Autodesk Inventor part; units mm, degrees
ref_plane "YZ Plane" through (0, 0, 0) normal (1, 0, 0) x (0, 1, 0)
ref_plane "XZ Plane" through (0, 0, 0) normal (0, 1, 0) x (-1, 0, 0)
ref_plane "XY Plane" through (0, 0, 0) normal (0, 0, 1) x (1, 0, 0)
sketch "Sketch1" plane through (0, 0, 0) normal (0, 0, 1) x (1, 0, 0)
  line L0 (0, 0) -> (75, 0)
  line L1 (75, 0) -> (75, 150)
  line L2 (75, 150) -> (0, 150)
  line L3 (0, 150) -> (0, 0)
  dimension "d0" = 75
  dimension "d1" = 150
extrude "Extrusion1" add sketch "Sketch1" along normal blind 10
sketch "Sketch2" plane through (0, 0, 10) normal (0, 0, 1) x (1, 0, 0)
  line L0 (17, 90) -> (17, 14)
  line L1 (17, 14) -> (27, 14)
  line L2 (27, 14) -> (27, 19)
  line L3 (27, 19) -> (22, 19)
  line L4 (22, 19) -> (22, 85)
  line L5 (22, 85) -> (27, 85)
  line L6 (27, 85) -> (27, 90)
  line L7 (27, 90) -> (17, 90)
  line L8 (75, 0) -> (75, 150)
  line L9 (75, 150) -> (0, 150)
  point P0 (0, 0)
  dimension "d4" = 76
  dimension "d5" = 10
  dimension "d6" = 5
  dimension "d7" = 66
  dimension "d8" = 53
  dimension "d9" = 5
  dimension "d10" = 60
extrude "Extrusion2" add sketch "Sketch2" along normal blind 5
sketch "Sketch3" plane through (22, 19, 10) normal (1, 0, 0) x (0, 0, -1)
  line L0 (-5, 0) -> (-5, 66)
  line L1 (-5, 66) -> (-3, 66)
  line L2 (-3, 66) -> (-3, 56)
  line L3 (-3, 56) -> (-5, 56)
  line L4 (-5, 56) -> (-5, 66)
  line L5 (-5, 0) -> (-3, 0)
  line L6 (-3, 0) -> (-3, 10)
  line L7 (-3, 10) -> (-5, 10)
  line L8 (-5, 10) -> (-5, 0)
  point P0 (10, -19)
  point P1 (-5, 10)
  point P2 (-5, 56)
  dimension "d13" = 2
  dimension "d14" = 10
  dimension "d15" = 10
  dimension "d73" = 2
extrude "Extrusion3" add sketch "Sketch3" along normal blind 3
sketch "Sketch4" plane through (0, 0, 10) normal (0, 0, 1) x (1, 0, 0)
  line L0 (75, 0) -> (75, 150)
  line L1 (75, 140) -> (10, 140)
  line L2 (10, 140) -> (10, 10)
  line L3 (10, 10) -> (75, 10)
  line L4 (75, 150) -> (0, 150)
  line L5 (0, 150) -> (0, 0)
  line L6 (0, 0) -> (75, 0)
  dimension "d18" = 10
  dimension "d19" = 10
  dimension "d20" = 10
extrude "Extrusion4" add sketch "Sketch4" along normal blind 140 contours L6 L5 L4 L0 L1 L2 L3
sketch "Sketch5" plane through (0, 0, 0) normal (-1, 0, 0) x (0, 0, 1)
  line L0 (90.0447, 124.5126) -> (90.0447, 94.5126)
  line L1 (90.0447, 94.5126) -> (109.0447, 94.5126)
  line L2 (109.0447, 94.5126) -> (109.0447, 64.5126)
  line L3 (109.0447, 64.5126) -> (90.0447, 64.5126)
  line L4 (90.0447, 64.5126) -> (90.0447, 77.5126)
  line L5 (90.0447, 77.5126) -> (76.4377, 86.2941)
  line L6 (76.4377, 86.2941) -> (46.4377, 86.2941)
  line L7 (46.4377, 86.2941) -> (46.4377, 56.2941)
  line L8 (46.4377, 56.2941) -> (65.4377, 56.2941)
  line L9 (65.4377, 56.2941) -> (65.4377, 37.2941)
  line L10 (65.4377, 37.2941) -> (77.4951, 29.5126)
  line L11 (77.4951, 29.5126) -> (118.4951, 29.5126)
  line L12 (118.4951, 29.5126) -> (135, 48.5)
  line L13 (135, 48.5) -> (135, 111.5)
  line L14 (135, 111.5) -> (120.0447, 124.5)
  line L15 (120.0447, 124.5) -> (90.0447, 124.5126)
  line L16 (0, 0) -> (150, 0)
  line L17 (150, 150) -> (150, 0)
  line L18 (36.4377, 86) -> (17.4377, 86)
  line L19 (17.4377, 86) -> (17.4377, 56)
  line L20 (17.4377, 56) -> (36.4377, 56)
  line L21 (36.4377, 56) -> (36.4377, 86)
  line L22 (10, 140) -> (150, 140)
  circle A0 centre (140, 140) radius 7.5
  line L23 (10, 10) -> (150, 10)
  circle A1 centre (140, 10) radius 7.5
  circle A2 centre (10, 140) radius 7.5
  line L24 (10, 10) -> (10, 140)
  circle A3 centre (10, 10) radius 7.5
  point P0 (99.5447, 64.5126)
  point P1 (135, 80)
  point P2 (26.9377, 56)
  dimension "d43" = 30
  dimension "d44" = 19
  dimension "d45" = 30
  dimension "d46" = 13
  dimension "d47" = 30
  dimension "d48" = 30
  dimension "d49" = 19
  dimension "d50" = 19
  dimension "d51" = 41
  dimension "d52" = 63
  dimension "d53" = 13
  dimension "d56" = 35
  dimension "d57" = 95
  dimension "d58" = 30
  dimension "d59" = 80
  dimension "d60" = 25.9553
  dimension "d61" = 15
  dimension "d62" = 19
  dimension "d63" = 10
  dimension "d67" = 15
  dimension "d68" = 15
  dimension "d69" = 15
  dimension "d70" = 15
  dimension "d71" = 10
  dimension "d72" = 10
  dimension "d112" = 56
  dimension "d113" = 30
extrude "Extrusion5" add sketch "Sketch5" along normal blind 3 contours L15 L14 L13 L12 L11 L10 L9 L8 L7 L6 L5 L4 L3 L2 L1 L0 | A0 L22 | L22 A0 | A1 L23 | L23 A1 | A2 L24 L22 | L22 L24 A2 | A3 L24 L23 | L23 L24 A3 | L21 L20 L19 L18
sketch "Sketch8" plane through (10, 10, 10) normal (0, 1, 0) x (1, 0, 0)
  line L0 (65, 0) -> (65, -140)
  line L1 (65, -115) -> (15, -115)
  line L2 (15, -115) -> (15, -85)
  line L3 (15, -85) -> (65, -85)
  line L4 (65, -115) -> (65, -120)
  line L5 (65, -120) -> (10, -120)
  line L6 (10, -120) -> (10, -80)
  line L7 (10, -80) -> (65, -80)
  line L8 (-10, -140) -> (65, -140)
  point P0 (-10, 10)
  dimension "d74" = 30
  dimension "d75" = 50
  dimension "d76" = 5
  dimension "d77" = 55
  dimension "d78" = 40
  dimension "d111" = 20
extrude "Extrusion6" add sketch "Sketch8" along normal blind 10 contours L0 L3 L2 L1 L5 L6 L7
sketch "Sketch10" plane through (25, 10, 125) normal (0, 1, 0) x (1, 0, 0)
  line L0 (50, 30) -> (50, 0)
  line L1 (0, 30) -> (50, 30)
  line L2 (50, 0) -> (0, 0)
  line L3 (0, 0) -> (0, 30)
  line L4 (0, 30) -> (50, 30)
  line L5 (50, 30) -> (50, 0)
  point P0 (-25, 125)
extrude "Extrusion7" cut sketch "Sketch10" against normal blind 10
sketch "Sketch11" plane through (25, 0, 95) normal (1, 0, 0) x (0, 0, -1)
  line L0 (85, 10) -> (-55, 10)
  line L1 (-29.957, 10) -> (0.043, 10)
  line L2 (0.043, 10) -> (0.043, 13)
  line L3 (0.043, 13) -> (-29.957, 13)
  line L4 (-29.957, 13) -> (-29.957, 10)
  line L5 (-30, 20) -> (0, 20)
  line L6 (-30, 20) -> (0, 20)
  line L7 (0, 20) -> (0, 17)
  line L8 (0, 17) -> (-30, 17)
  line L9 (-30, 17) -> (-30, 20)
  point P0 (95, 0)
  dimension "d83" = 30
  dimension "d84" = 30
  dimension "d85" = 3
  dimension "d86" = 3
extrude "Extrusion8" add sketch "Sketch11" along normal blind 5
sketch "Sketch12" plane through (75, 0, 0) normal (1, 0, 0) x (0, 0, -1)
  circle A0 centre (-5, 30) radius 2.5
  circle A1 centre (-5, 120) radius 2.5
  circle A2 centre (-120, 145) radius 2.5
  circle A3 centre (-30, 145) radius 2.5
  circle A4 centre (-60, 5) radius 2.5
  line L0 (-150, 140) -> (-150, 150)
  line L1 (0, 150) -> (-150, 150)
  line L2 (0, 0) -> (0, 150)
  line L3 (0, 0) -> (-95, 0)
  line L4 (-10, 10) -> (-90, 10)
  point P0 (-150, 145)
  dimension "d89" = 5
  dimension "d90" = 5
  dimension "d91" = 5
  dimension "d92" = 5
  dimension "d93" = 5
  dimension "d94" = 30
  dimension "d95" = 5
  dimension "d96" = 30
  dimension "d97" = 5
  dimension "d98" = 5
  dimension "d99" = 30
  dimension "d100" = 30
  dimension "d101" = 5
  dimension "d102" = 5
  dimension "d103" = 60
sketch "Sketch13" plane through (0, 0, 0) normal (0, -1, 0) x (1, 0, 0)
  circle A0 centre (38, 40) radius 10
  line L0 (75, 0) -> (75, 95)
  line L1 (0, 0) -> (75, 0)
  point P0 (37.5, 0)
  dimension "d106" = 20
  dimension "d107" = 37
  dimension "d108" = 40
extrude "Extrusion9" add sketch "Sketch12" along normal blind 5
extrude "Extrusion10" cut sketch "Sketch13" against normal blind 10
properties part number "vraagblok"
Design review of the part built by this model. Coordinates are the model's own, in mm. A direction names the side the tool comes from. Coordinates: 2 decimals unless noted, no trailing zeros. Order: outer loops, then holes, each group sorted by start corner. A loop starts at its lowest first (then second) coordinate and runs counter-clockwise, first axis right, second up. Notation, with made-up numbers: (49, -38) - (57, -38) arc R36 ccw to (57, -1) - close; hole circle Ø10 at (14, 16). An arc over 180 degrees is marked (long way). One line per question, with ' | ' between items.
Q1. For faces 1 (the flat face through (43, 140, 79)), 2 (the flat face through (22, 14, 12)), 3 (the cylindrical face through (-1.48, 12.87, 146.93)), list the 3-axis set-ups (+Z, -Z, +X, -X, +Y, -Y) from which the entire face can be reached by the end or side of a thin tool; tool diameter is ignored.
Answer key:
face 1: +Z, +X | face 2: +X | face 3: -X
Q2. Consider section C-C, the plane y = 5. Give the boundary of the cut face in (x, z).
Answer key:
outline: (-3, 4.41) - (0, 4.41) - (0, 0) - (75, 0) - (75, 57.5) - (80, 57.5) - (80, 62.5) - (75, 62.5) - (75, 95) - (25, 95) - (25, 125) - (75, 125) - (75, 150) - (0, 150) - (0, 145.59) - (-3, 145.59) - (-3, 134.41) - (0, 134.41) - (0, 15.59) - (-3, 15.59) - close; hole circle Ø20 at (38, 40)
Q3. The part is to be moulded in two halves that separate along Z. For faces 4 (the flat face through (-3, 10, 10)), 5 (the cylindrical face through (77.46, 5.96, 57.69)), 6 (the flat face through (50, 10, 95)), say which applies: +Z half, -Z half, draft (parallel to the pull), parting line (faces both ways), or undercut.
Answer key:
face 4: draft | face 5: parting line | face 6: undercut
Q4. Consider section D-D, the plane z = 60. Give the boundary of the cut face in (x, y).
Answer key:
outline: (-3, 56.29) - (0, 56.29) - (0, 0) - (75, 0) - (75, 2.5) - (80, 2.5) - (80, 7.5) - (75, 7.5) - (75, 10) - (10, 10) - (10, 140) - (75, 140) - (75, 150) - (0, 150) - (0, 86.29) - (-3, 86.29) - close
Q5. To check wall thickness, follow line 1 along Z through (x, y) = (38, 3); line 2 along Y through (x, z) = (29.5, 128); line 3 along Y through (x, z) = (19, 51). State the ranges of each line that lie inside material, in increasing order.
Answer key:
line 1: z = 0 to 30, 50 to 95, 125 to 150 | line 2: y = 0 to 20, 140 to 150 | line 3: y = 0 to 10, 140 to 150
Q6. Clearance check with flat-ended pins moving along their axes: pin 1 Ø0.9 at (x, y) = (-2, 69.5) entering from +Z; pin 2 Ø3 at (y, z) = (13, 117.5) entering from -X; pin 3 Ø2 at (y, z) = (51, 68) entering from +X. State where each tip first meets the part, or that it passes through.
Answer key:
pin 1: stops at z = 135 | pin 2: stops at x = 0 | pin 3: stops at x = 10
Q7. Consider section B-B, the plane y = 68. Give the boundary of the cut face in (x, z).
Answer key:
outline: (-3, 17.44) - (0, 17.44) - (0, 0) - (75, 0) - (75, 10) - (22, 10) - (22, 15) - (17, 15) - (17, 10) - (10, 10) - (10, 150) - (0, 150) - (0, 135) - (-3, 135) - (-3, 109.04) - (0, 109.04) - (0, 90.04) - (-3, 90.04) - (-3, 46.44) - (0, 46.44) - (0, 36.44) - (-3, 36.44) - close
Q8. Consider section A-A, the plane z = 40. Give the boundary of the cut face in (x, y), then the cut area to 3 significant figures.
Answer key:
outline: (0, 0) - (28, 0) - (28, 10) - (10, 10) - (10, 140) - (75, 140) - (75, 150) - (0, 150) - close; (48, 0) - (75, 0) - (75, 10) - (48, 10) - close | area: 2,600 mm2
